```python
from build123d import *

# Parameters (mm, degrees)
SKETCH1_W                      = 170
SKETCH1_H                      = 70
BOSS_EXTRUDE1_DEPTH            = 4
SKETCH2_W                      = 159
SKETCH2_H                      = 50
BOSS_EXTRUDE2_DEPTH            = 4
M3_CLEARANCE_HOLE1_D           = 3.4
M3_CLEARANCE_HOLE1_CSINK_D     = 3.5
M3_CLEARANCE_HOLE1_CSINK_ANGLE = 90
SKETCH6_R                      = 1.75
SKETCH6_W                      = 18
SKETCH6_H                      = 8.5
SKETCH6_W_2                    = 22
SKETCH6_H_2                    = 28.7
SKETCH6_W_3                    = 7
SKETCH6_H_3                    = 15
CUT_EXTRUDE1_DEPTH             = 9
CUT_EXTRUDE2_START             = -8
SKETCH6_3_W                    = 18
SKETCH6_3_H                    = 8.5
SKETCH6_3_W_2                  = 32.5
SKETCH6_3_H_2                  = 12.8
CUT_EXTRUDE2_DEPTH             = 3
CHAMFER1_SIZE                  = 1
FILLET1_R                      = 5


with BuildPart() as part:
    # Sketch1 → Boss-Extrude1 (new body)
    with BuildSketch(Plane(origin=(0, 0, 0), x_dir=(1, 0, 0), z_dir=(0, 1, 0))):
        Rectangle(SKETCH1_W, SKETCH1_H)
    extrude(amount=BOSS_EXTRUDE1_DEPTH)

    # Sketch2 → Boss-Extrude2 (add)
    with BuildSketch(Plane(origin=(0, 4, 0), x_dir=(1, 0, 0), z_dir=(0, 1, 0))):
        Rectangle(SKETCH2_W, SKETCH2_H)
    extrude(amount=BOSS_EXTRUDE2_DEPTH)

    # M3 Clearance Hole1 (through all)
    with Locations(Plane(origin=(0, 4, 0), x_dir=(1, 0, 0), z_dir=(0, 1, 0))):
        with Locations((80.5, -30.5), (80.5, 30.5), (-80.5, -30.5), (-80.5, 30.5)):
            CounterSinkHole(M3_CLEARANCE_HOLE1_D / 2, M3_CLEARANCE_HOLE1_CSINK_D / 2, counter_sink_angle=M3_CLEARANCE_HOLE1_CSINK_ANGLE)

    # Sketch6 → Cut-Extrude1 (cut, through all)
    with BuildSketch(Plane.XZ):
        with Locations((-48, 0)):
            Circle(SKETCH6_R)
        with Locations((-73, 0)):
            Circle(SKETCH6_R)
        with Locations((-60.5, 0)):
            Rectangle(SKETCH6_W, SKETCH6_H)
        with Locations((-33.75, 10.8)):
            Circle(SKETCH6_R)
        with Locations((-33.75, -10.8)):
            Circle(SKETCH6_R)
        with Locations((-14.75, 10.8)):
            Circle(SKETCH6_R)
        with Locations((-14.75, -10.8)):
            Circle(SKETCH6_R)
        Circle(SKETCH6_R)
        with Locations((58.5, 0)):
            Rectangle(SKETCH6_W_2, SKETCH6_H_2)
        with Locations((-33.75, 0)):
            Rectangle(SKETCH6_W_3, SKETCH6_H_3)
        with Locations((-14.75, 0)):
            Rectangle(SKETCH6_W_3, SKETCH6_H_3)
        Polygon((28, 9.5), (34, 5.894448725), (34, -9.5), (6, -9.5), (6, 5.894448725), (12, 9.5), align=None)
        with Locations((40, 0)):
            Circle(SKETCH6_R)
    extrude(amount=-CUT_EXTRUDE1_DEPTH, mode=Mode.SUBTRACT)

    # Sketch6<3> → Cut-Extrude2 (cut)
    with BuildSketch(Plane.XZ.offset(CUT_EXTRUDE2_START)):
        with Locations((-60.5, 0)):
            Rectangle(SKETCH6_3_W, SKETCH6_3_H)
        with Locations((-60.5, 0)):
            Rectangle(SKETCH6_3_W_2, SKETCH6_3_H_2)
    extrude(amount=CUT_EXTRUDE2_DEPTH, mode=Mode.SUBTRACT)

    # Chamfer1
    chamfer1_edges = [part.edges().sort_by_distance(p)[0] for p in [
        (69.5, 0, 0),
        (58.5, 0, 14.35),
        (47.5, 0, 0),
        (58.5, 0, -14.35),
        (-37.25, 0, 0),
        (-33.75, 0, 7.5),
        (-33.75, 0, -7.5),
        (-30.25, 0, 0),
        (-18.25, 0, 0),
        (-14.75, 0, 7.5),
        (-14.75, 0, -7.5),
        (-11.25, 0, 0),
        (20, 0, 9.5),
        (31, 0, 7.697224362),
        (34, 0, -1.802775638),
        (20, 0, -9.5),
        (9, 0, 7.697224362),
        (6, 0, -1.802775638),
        (-79.5, 8, 0),
        (0, 8, -25),
        (0, 8, 25),
        (79.5, 8, 0),
        (-51.5, 0, 0),
        (-60.5, 0, 4.25),
        (-69.5, 0, 0),
        (-60.5, 0, -4.25),
    ]]
    chamfer(chamfer1_edges, length=CHAMFER1_SIZE)

    # Fillet1
    fillet1_edges = [part.edges().sort_by_distance(p)[0] for p in [
        (85, 2, 35),
        (-85, 2, 35),
        (-85, 2, -35),
        (85, 2, -35),
    ]]
    fillet(fillet1_edges, radius=FILLET1_R)


solid = part.part
```
Read the model definition and answer for the solid it produces. Units are mm, in the model's axes. A direction names the side the tool comes from. Round coordinates to 2 decimals unless told otherwise and drop trailing zeros. Loops run counter-clockwise (first coordinate to the right, second up) from the corner with the lowest first, then second, coordinate; pieces in that order, holes last. Notation, with made-up numbers: (-15, 35.5) -> (7, 35.5) arc R22 ccw to (7, 64.5) -> close; hole circle Ø3 at (-15.5, 2.5). An arc over 180 degrees is marked (long way). One line per item, written item: value.
1) Consider L1, parallel to Z at x = 80.5, y = 1.95; L2, parallel to X at y = 1.3, z = 30.5; L3, parallel to Z at x = 40, y = 5.25. Determine where each line is inside the solid, lowest interval first. Write a range as [from, to].
Answer list:
L1: z = [-34.97, -32.2], [-28.8, 28.8], [32.2, 34.97]
L2: x = [-84.97, -82.2], [-78.8, 78.8], [82.2, 84.97]
L3: z = [-25, -1.75], [1.75, 25]
2) A cutting plane is placed at C-C (z = 0). Give the number of separate pieces and of enclosed holes in the cut face, and give its area (4 significant figures).
Answer list:
separate pieces: 10
enclosed holes: 0
area: 519.5 mm²
3) A cutting plane is placed at D-D (x = 40). Determine the outline of the cut face in (y, z), and give its area (3 significant figures).
Answer list:
outline: (0, -35) -> (4, -35) -> (4, -25) -> (7, -25) -> (8, -24) -> (8, -1.75) -> (0, -1.75) -> close; (0, 1.75) -> (8, 1.75) -> (8, 24) -> (7, 25) -> (4, 25) -> (4, 35) -> (0, 35) -> close
area: 451 mm²
4) For faces 4 (the face through (20, 4, 9.5)), 5 (the face through (-1, 2, 35)), 6 (the face through (-44.25, 7, 0)), determine the directions among +Z, -Z, +X, -X, +Y, -Y from which every point of the face is accessible in a straight line to the end or side of a thin tool.
Answer list:
face 4: +Y, -Y
face 5: +Z, +X, -X, +Y, -Y
face 6: +Y
5) A cutting plane is placed at A-A (x = 14). Determine the outline of the cut face in (y, z).
Answer list:
outline: (0, -35) -> (4, -35) -> (4, -25) -> (7, -25) -> (8, -24) -> (8, -9.5) -> (1, -9.5) -> (0, -10.5) -> close; (0, 10.5) -> (1, 9.5) -> (8, 9.5) -> (8, 24) -> (7, 25) -> (4, 25) -> (4, 35) -> (0, 35) -> close
6) The mould has two halves that part along Z. Classify faces 1 (the face through (-18.25, 4, 0)), 2 (the face through (83, 2, -34)), 3 (the face through (-1, 5, 25)): pulls with the +Z half, pulls with the -Z half, needs draft (parallel to the pull), parting line crosses it, or undercut.
Answer list:
face 1: undercut
face 2: pulls with the -Z half
face 3: pulls with the +Z half
7) A cutting plane is placed at B-B (x = -14.75). Determine the outline of the cut face in (y, z), and give its area (3 significant figures).
Answer list:
outline: (0, -35) -> (4, -35) -> (4, -25) -> (7, -25) -> (8, -24) -> (8, -12.55) -> (0, -12.55) -> close; (0, -9.05) -> (8, -9.05) -> (8, -7.5) -> (1, -7.5) -> (0, -8.5) -> close; (0, 8.5) -> (1, 7.5) -> (8, 7.5) -> (8, 9.05) -> (0, 9.05) -> close; (0, 12.55) -> (8, 12.55) -> (8, 24) -> (7, 25) -> (4, 25) -> (4, 35) -> (0, 35) -> close
area: 302 mm²
8) Flat-ended cylindrical pins translate along their axes: P1, Ø2, axis at x = -33.75, z = 10.8, coming from the +Y side; P2, Ø2.5, axis at x = 20, y = 5.5, coming from the +Z side; P3, Ø0.9, axis at y = 6, z = 2.5, coming from the -X side. Find the tip coordinate at first contact, or state that the pin passes through.
Answer list:
P1: passes through
P2: stops at z = 25
P3: stops at x = -79.5
